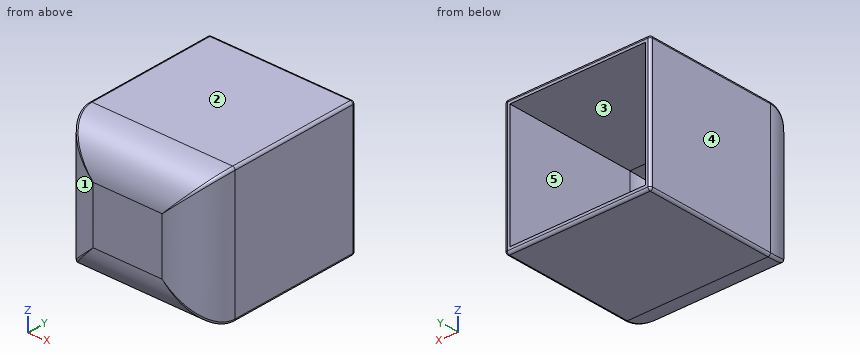
from build123d import *

# Parameters (mm, degrees)
F0_W     = 57
F0_H     = 52
F1_DEPTH = 67
F2_R     = 15
F3_T     = -2
F4_R     = 1
F5_R     = 1
F6_R     = 1


with BuildPart() as f1:
    # F0 (on Front) → F1 (new body)
    with BuildSketch(Plane.XZ):
        Rectangle(F0_W, F0_H)
    extrude(amount=F1_DEPTH)

    # F2
    f2_edges = [f1.edges().sort_by_distance(p)[0] for p in [
        (0, -67, 26),
        (-28.5, -67, 0),
        (0, -67, -26),
        (28.5, -67, 0),
    ]]
    fillet(f2_edges, radius=F2_R)

    # F3
    f3_openings = [f1.faces().sort_by_distance(p)[0] for p in [
        (0, 0, 0),
    ]]
    offset(amount=F3_T, openings=f3_openings)

    # F4
    f4_edges = [f1.edges().sort_by_distance(p)[0] for p in [
        (-28.5, 0, 0),
    ]]
    fillet(f4_edges, radius=F4_R)

    # F5
    f5_edges = [f1.edges().sort_by_distance(p)[0] for p in [
        (28.5, 0, 0),
    ]]
    fillet(f5_edges, radius=F5_R)

    # F6
    f6_edges = [f1.edges().sort_by_distance(p)[0] for p in [
        (28.5, -26.5, 26),
        (28.5, -26.5, -26),
        (-28.5, -26.5, 26),
        (-28.5, -26.5, -26),
    ]]
    fillet(f6_edges, radius=F6_R)


solid = f1.part
Can you work these out from the model? Positions are in its coordinate system, mm. Face numbers are marked on the shaded views. A direction names the side the tool comes from. Round coordinates to 2 decimals unless told otherwise and drop trailing zeros. Write each loop counter-clockwise with the first axis right and the second up, starting at its lowest first coordinate (ties: lowest second). Pieces come first, ordered by that corner, then holes. Notation, with made-up numbers: (14, -40) -> (54, -40) arc R20 ccw to (54, -17) -> close; hole circle Ø5 at (5.5, 64). An arc over 180 degrees is marked (long way). Use one line per item in the form item = value. Start each with the question number.
Q1. If I drill on probe 1 along X at (y, z) = (-6.5, 9.5); probe 2 along Z at (x, y) = (9.5, -29); probe 3 along X at (y, z) = (-58, 21.5), over which ranges is the centre line in solid material (lowest first)? Write a range as [from, to].
Q2. I'm going to push flat-ended pins straight in: P1, Ø17.5, axis at x = -3.5, z = 0.5, coming from the +Y side; P2, Ø1, axis at x = -18, z = -19.5, coming from the -Y side; P3, Ø5, axis at x = 2, z = 18, coming from the +Y side. Where does each tip first touch, or does it pass through?
Q3. We'd pull the mould along Z, two halves only. Please class the marked faces 1, 2 and 3: +Z half, -Z half, draft (parallel to the pull), parting line (faces both ways), or undercut.
Q4. Imagine slicing it at A-A (x = -7). Please give me the cut outline in (y, z), then the cut area to 3 significant figures.
Q5. Imagine slicing it at C-C (z = -2). Please give me the cut outline in (x, y), then the cut area to 3 significant figures.
Q6. Imagine slicing it at B-B (y = -42). Please give me the cut outline in (x, z), then the cut area to 3 significant figures.
Q7. Which directions (+Z, -Z, +X, -X, +Y, -Y) give clear straight access to the entire face, cutting with the end or side of a thin tool? Please do the marked faces 4 and 5.
Worked out:
q1.probe_1 = [-28.5, -26.5], [26.5, 28.5]
q1.probe_2 = [-26, -24], [24, 26]
q1.probe_3 = [-27.25, -25.03], [25.03, 27.25]
q2.P1 = -65
q2.P2 = -64.69
q2.P3 = -60.87
q3.face_1 = draft
q3.face_2 = +Z half
q3.face_3 = undercut
q4.outline = (-67, -11) arc R15 ccw to (-52, -26) -> (-1, -26) arc R1 ccw to (0, -25) -> (0, -24) -> (-52, -24) arc R13 cw to (-65, -11) -> (-65, 11) arc R13 cw to (-52, 24) -> (0, 24) -> (0, 25) arc R1 ccw to (-1, 26) -> (-52, 26) arc R15 ccw to (-67, 11) -> close
q4.area = 340 mm^2
q5.outline = (-28.5, -52) arc R15 ccw to (-13.5, -67) -> (13.5, -67) arc R15 ccw to (28.5, -52) -> (28.5, -1) arc R1 ccw to (27.5, 0) -> (26.5, 0) -> (26.5, -52) arc R13 cw to (13.5, -65) -> (-13.5, -65) arc R13 cw to (-26.5, -52) -> (-26.5, 0) -> (-27.5, 0) arc R1 ccw to (-28.5, -1) -> close
q5.area = 350 mm^2
q6.outline = (-28.5, -25) arc R1 ccw to (-27.5, -26) -> (27.5, -26) arc R1 ccw to (28.5, -25) -> (28.5, 25) arc R1 ccw to (27.5, 26) -> (-27.5, 26) arc R1 ccw to (-28.5, 25) -> close; hole (-26.5, -24) -> (26.5, -24) -> (26.5, 24) -> (-26.5, 24) -> close
q6.area = 419 mm^2
q7.face_4 = +Z, -Z, -X, +Y, -Y
q7.face_5 = +Y
